For this review, take the finished solid that the model builds, in its own axes (mm). Round coordinates to 2 decimals unless told otherwise and drop trailing zeros. Loops run counter-clockwise (first coordinate to the right, second up) from the corner with the lowest first, then second, coordinate; pieces in that order, holes last.
1) Take a section at A-A (x = 0). State the section outline as (y, z) points, then the cut area to 3 significant figures.
2) Insertion check: pin 1 (3 mm diameter, centred on y = 3, z = 1, fed in from -X); pin 2 (3 mm diameter, centred on x = -0.5, y = -0.5, fed in from +Z); pin 3 (1 mm diameter, centred on y = 3.5, z = 3.5, fed in from -X); pin 4 (1 mm diameter, centred on x = 0, y = -3, fed in from -Z). Each pin has a flat end and moves straight along its axis. Give the tip position at first contact, or say it passes through.
3) Take a section at C-C (z = 2.4). State the section outline as (x, y) points.
4) Mouldability with a two-part tool opening along Y and no side actions: class faces 1 (the flat face through (0, -1, 0)), 2 (the cylindrical face through (-3.047, 0.134, 3.028)), 3 (the cylindrical face through (-0.59, -4.46, 2.97)) as pulls with the +Y half, pulls with the -Y half, needs draft (parallel to the pull), parting line crosses it, or undercut.
5) Wall thickness on L1, parallel to Y at x = 0, z = 2.6; L2, parallel to Y at x = 0, z = 0.2; L3, parallel to Z at x = 0.25, y = 1.5: over which ranges is each line inside the solid? List them lowest first.
Autodesk Inventor part; units mm, degrees
ref_plane "YZ Plane" through (0, 0, 0) normal (1, 0, 0) x (0, 1, 0)
ref_plane "XZ Plane" through (0, 0, 0) normal (0, 1, 0) x (-1, 0, 0)
ref_plane "XY Plane" through (0, 0, 0) normal (0, 0, 1) x (1, 0, 0)
sketch "Sketch1" plane through (0, 0, 0) normal (0, 0, 1) x (1, 0, 0)
  circle A0 centre (0, 0) radius 4.5
  dimension "d0" = 9
extrude "Extrusion1" add sketch "Sketch1" along normal blind 5
sketch "Sketch2" plane through (0, 0, 5) normal (0, 0, 1) x (1, 0, 0)
  circle A0 centre (0, 0) radius 3.05
  dimension "d3" = 6.1
extrude "Extrusion2" cut sketch "Sketch2" against normal blind 4
chamfer "Chamfer1" distance 1 angle 45 1 edges at (-4.5, 0, 0)
sketch "Sketch3" plane through (0, 0, 1) normal (0, 0, 1) x (1, 0, 0)
  circle A0 centre (0, 0) radius 0.25
  dimension "d9" = 0.5
extrude "Extrusion3" cut sketch "Sketch3" against normal through all
fillet "Fillet1" radius 0.5 1 edges at (-0.25, 0, 1)
properties part number "laser_diode_lid"
Response:
1. outline: (-4.5, 1) - (-3.5, 0) - (-0.25, 0) - (-0.25, 0.5) arc R0.5 ccw to (-0.75, 1) - (-3.05, 1) - (-3.05, 5) - (-4.5, 5) - close; (0.25, 0) - (3.5, 0) - (4.5, 1) - (4.5, 5) - (3.05, 5) - (3.05, 1) - (0.75, 1) arc R0.5 ccw to (0.25, 0.5) - close
1. area: 19.0 mm2
2. pin 1: stops at x = -4.24
2. pin 2: stops at z = 1
2. pin 3: stops at x = -3.35
2. pin 4: stops at z = 0
3. outline: circle Ø9 at (0, 0); hole circle Ø6.1 at (0, 0)
4. face 1: needs draft
4. face 2: undercut
4. face 3: parting line crosses it
5. L1: y = -4.5 to -3.05, 3.05 to 4.5
5. L2: y = -3.7 to -0.25, 0.25 to 3.7
5. L3: z = 0 to 1
